Source: CAD feature listing. Evaluate the final solid. Frame: model axes, mm. Face numbers are marked on the shaded views. Give positions to 0.01 mm unless a question says otherwise; leave off trailing zeros. Order: outer loops, then holes, each group sorted by start corner. A loop starts at its lowest first (then second) coordinate and runs counter-clockwise, first axis right, second up. Notation, with made-up numbers: (66.5, 22.25) -> (121.5, 22.25) arc R21 ccw to (121.5, 30.25) -> close; hole circle Ø8 at (71.5, 57.5). An arc over 180 degrees is marked (long way). Answer in a Markdown table with one row per item.
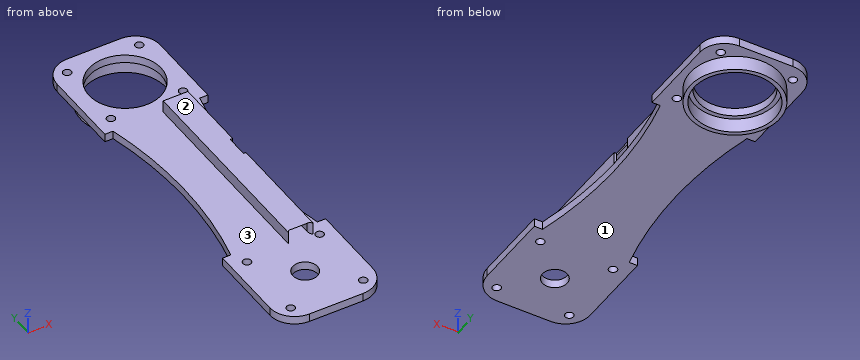
```python
from build123d import *

# Parameters (mm, degrees)
SKETCH1_R           = 11.1125
SKETCH1_R_2         = 1.27
BOSS_EXTRUDE1_DEPTH = 2.54
SKETCH2_R           = 1.27
SKETCH2_R_2         = 3.81
CUT_EXTRUDE1_DEPTH  = 2.54
SKETCH3_R           = 13.716
SKETCH3_R_2         = 12.446
BOSS_EXTRUDE2_DEPTH = 4.445
SKETCH4_W           = 7.62
SKETCH4_H           = 64.008
SKETCH4_W_2         = 6.096
SKETCH4_H_2         = 62.484
EXTRUDE_THIN1_DEPTH = 3.81
SKETCH5_W           = 6.096
SKETCH5_H           = 3.81
CUT_EXTRUDE2_DEPTH  = 76.2
SKETCH6_W           = 7.62
SKETCH6_H           = 64.008
BOSS_EXTRUDE3_DEPTH = 0.762
FILLET1_R           = 2.54
SKETCH7_W           = 3.81
SKETCH7_H           = 6.858
CUT_EXTRUDE3_DEPTH  = 0.762


with BuildPart() as part:
    # Sketch1 → Boss-Extrude1 (new body)
    with BuildSketch(Plane.XY):
        with BuildLine():
            Line((-13.335, -76.2), (-15.875, -76.2))
            Line((-15.875, -76.2), (-15.875, -100.33))
            ThreePointArc((-15.875, -100.33), (-13.643153673, -105.718153673), (-8.255, -107.95))
            Line((-8.255, -107.95), (8.255, -107.95))
            ThreePointArc((8.255, -107.95), (13.643153673, -105.718153673), (15.875, -100.33))
            Line((15.875, -100.33), (15.875, -76.2))
            Line((15.875, -76.2), (13.335, -76.2))
            ThreePointArc((13.335, -76.2), (9.716725547, -46.101), (13.335, -16.002))
            Line((13.335, -16.002), (15.875, -16.002))
            Line((15.875, -16.002), (15.875, 8.382))
            ThreePointArc((15.875, 8.382), (13.643153673, 13.770153673), (8.255, 16.002))
            Line((8.255, 16.002), (-8.255, 16.002))
            ThreePointArc((-8.255, 16.002), (-13.643153673, 13.770153673), (-15.875, 8.382))
            Line((-15.875, 8.382), (-15.875, -16.002))
            Line((-15.875, -16.002), (-13.335, -16.002))
            ThreePointArc((-13.335, -16.002), (-9.716725547, -46.101), (-13.335, -76.2))
        make_face()
        Circle(SKETCH1_R, mode=Mode.SUBTRACT)
        with Locations((11.1125, 11.2014)):
            Circle(SKETCH1_R_2, mode=Mode.SUBTRACT)
        with Locations((11.1125, -11.2014)):
            Circle(SKETCH1_R_2, mode=Mode.SUBTRACT)
        with Locations((-11.1125, -11.2014)):
            Circle(SKETCH1_R_2, mode=Mode.SUBTRACT)
        with Locations((-11.1125, 11.2014)):
            Circle(SKETCH1_R_2, mode=Mode.SUBTRACT)
    extrude(amount=BOSS_EXTRUDE1_DEPTH)

    # Sketch2 → Cut-Extrude1 (cut)
    with BuildSketch(Plane(origin=(0, 0, 0), x_dir=(-1, 0, 0), z_dir=(0, 0, -1))):
        with Locations((-11.176, -80.899)):
            Circle(SKETCH2_R)
        with Locations((11.176, -80.899)):
            Circle(SKETCH2_R)
        with Locations((11.176, -103.251)):
            Circle(SKETCH2_R)
        with Locations((-11.176, -103.251)):
            Circle(SKETCH2_R)
        with Locations((0, -92.075)):
            Circle(SKETCH2_R_2)
    extrude(amount=-CUT_EXTRUDE1_DEPTH, mode=Mode.SUBTRACT)

    # Sketch3 → Boss-Extrude2 (add)
    with BuildSketch(Plane(origin=(0, 0, 0), x_dir=(-1, 0, 0), z_dir=(0, 0, -1))):
        with Locations(Location((0, 0, 0), (0, 0, 180))):
            Circle(SKETCH3_R)
        Circle(SKETCH3_R_2, mode=Mode.SUBTRACT)
    extrude(amount=BOSS_EXTRUDE2_DEPTH)

    # Sketch4 → Extrude-Thin1 (add)
    with BuildSketch(Plane.XY.offset(2.54)):
        with Locations((5.906725547, -48.006)):
            Rectangle(SKETCH4_W, SKETCH4_H)
        with Locations((5.906725547, -48.006)):
            Rectangle(SKETCH4_W_2, SKETCH4_H_2, mode=Mode.SUBTRACT)
    extrude(amount=EXTRUDE_THIN1_DEPTH)

    # Sketch5 → Cut-Extrude2 (cut)
    with BuildSketch(Plane.XZ.offset(80.01)):
        with Locations((5.906725547, 4.445)):
            Rectangle(SKETCH5_W, SKETCH5_H)
    extrude(amount=-CUT_EXTRUDE2_DEPTH, mode=Mode.SUBTRACT)

    # Sketch6 → Boss-Extrude3 (add)
    with BuildSketch(Plane.XY.offset(6.35)):
        with Locations((5.906725547, -48.006)):
            Rectangle(SKETCH6_W, SKETCH6_H)
    extrude(amount=-BOSS_EXTRUDE3_DEPTH)

    # Fillet1
    # the kernel refuses this fillet: 2.54 mm, written as the material it takes off along each edge
    with BuildSketch(Plane(origin=(8.954725547, -80.01, 5.588), x_dir=(0, 1, 0), z_dir=(0, 0, -1)), Plane(origin=(2.858725547, -80.01, 2.54), x_dir=(0, 1, 0), z_dir=(0, 0, 1))) as fillet1_piece_1:
        with BuildLine():
            CenterArc((1.813922821, 2.54), FILLET1_R, 224.427004001, 45.572995999)
            Line((0, 0.762), (0, 0))
            Line((0, 0), (1.813922821, 0))
        make_face()
    extrude(amount=3.048, mode=Mode.SUBTRACT)
    with BuildSketch(Plane(origin=(8.954725547, -80.01, 5.588), x_dir=(0, 1, 0), z_dir=(-1, 0, 0))) as fillet1_piece_2:
        with BuildLine():
            CenterArc((FILLET1_R, -FILLET1_R), FILLET1_R, 90, 90)
            Line((0, -FILLET1_R), (0, 0))
            Line((0, 0), (FILLET1_R, 0))
        make_face()
    extrude(amount=6.096, mode=Mode.SUBTRACT)
    with BuildSketch(Plane(origin=(15.304725547, -80.01, 5.588), x_dir=(0, 1, 0), z_dir=(-1, 0, 0))) as fillet1_piece_3a_section:
        with BuildLine():
            CenterArc((FILLET1_R, -FILLET1_R), FILLET1_R, 90, 90)
            Line((0, -FILLET1_R), (0, 0))
            Line((0, 0), (FILLET1_R, 0))
        make_face()
    fillet1_piece_3a = extrude(amount=12.446, mode=Mode.PRIVATE)
    fillet1_piece_3a = split(fillet1_piece_3a, bisect_by=Plane(origin=(15.304725547, -80.01, 6.35), z_dir=(0, 0, -1)), keep=Keep.TOP, mode=Mode.PRIVATE)
    fillet1_piece_3a = split(fillet1_piece_3a, bisect_by=Plane(origin=(8.954725547, -80.01, 5.588), z_dir=(1, 0, 0)), keep=Keep.TOP, mode=Mode.PRIVATE)
    fillet1_piece_3a = split(fillet1_piece_3a, bisect_by=Plane(origin=(9.716725547, -80.01, 5.588), z_dir=(-1, 0, 0)), keep=Keep.TOP, mode=Mode.PRIVATE)
    with BuildSketch(Plane(origin=(8.954725547, -80.01, 10.122807052), x_dir=(0, 1, 0), z_dir=(0, 0, -1))) as fillet1_piece_3b_section:
        with BuildLine():
            CenterArc((1.813922821, 2.54), FILLET1_R, 224.427004001, 45.572995999)
            Line((0, 0.762), (0, 0))
            Line((0, 0), (1.813922821, 0))
        make_face()
    fillet1_piece_3b = extrude(amount=7.582807052, mode=Mode.PRIVATE)
    fillet1_piece_3b = split(fillet1_piece_3b, bisect_by=Plane(origin=(8.954725547, -80.01, 6.35), z_dir=(0, 0, -1)), keep=Keep.TOP, mode=Mode.PRIVATE)
    fillet1_piece_3b = split(fillet1_piece_3b, bisect_by=Plane(origin=(8.954725547, -80.01, 5.588), z_dir=(0, 0, 1)), keep=Keep.TOP, mode=Mode.PRIVATE)
    fillet1_piece_3 = fillet1_piece_3a & fillet1_piece_3b
    add(fillet1_piece_3, mode=Mode.SUBTRACT)
    with BuildSketch(Plane(origin=(2.858725547, -80.01, 2.54), x_dir=(0, 1, 0), z_dir=(0, 0, 1))) as fillet1_piece_4a_section:
        with BuildLine():
            CenterArc((1.813922821, 2.54), FILLET1_R, 224.427004001, 45.572995999)
            Line((0, 0.762), (0, 0))
            Line((0, 0), (1.813922821, 0))
        make_face()
    fillet1_piece_4a = extrude(amount=7.582807052, mode=Mode.PRIVATE)
    fillet1_piece_4a = split(fillet1_piece_4a, bisect_by=Plane(origin=(2.858725547, -80.01, 6.35), z_dir=(0, 0, -1)), keep=Keep.TOP, mode=Mode.PRIVATE)
    fillet1_piece_4a = split(fillet1_piece_4a, bisect_by=Plane(origin=(2.858725547, -80.01, 5.588), z_dir=(0, 0, 1)), keep=Keep.TOP, mode=Mode.PRIVATE)
    with BuildSketch(Plane(origin=(8.954725547, -80.01, 5.588), x_dir=(0, 1, 0), z_dir=(-1, 0, 0))) as fillet1_piece_4b_section:
        with BuildLine():
            CenterArc((FILLET1_R, -FILLET1_R), FILLET1_R, 90, 90)
            Line((0, -FILLET1_R), (0, 0))
            Line((0, 0), (FILLET1_R, 0))
        make_face()
    fillet1_piece_4b = extrude(amount=12.446, mode=Mode.PRIVATE)
    fillet1_piece_4b = split(fillet1_piece_4b, bisect_by=Plane(origin=(2.096725547, -80.01, 5.588), z_dir=(1, 0, 0)), keep=Keep.TOP, mode=Mode.PRIVATE)
    fillet1_piece_4b = split(fillet1_piece_4b, bisect_by=Plane(origin=(8.954725547, -80.01, 6.35), z_dir=(0, 0, -1)), keep=Keep.TOP, mode=Mode.PRIVATE)
    fillet1_piece_4b = split(fillet1_piece_4b, bisect_by=Plane(origin=(2.858725547, -80.01, 5.588), z_dir=(-1, 0, 0)), keep=Keep.TOP, mode=Mode.PRIVATE)
    fillet1_piece_4 = fillet1_piece_4a & fillet1_piece_4b
    add(fillet1_piece_4, mode=Mode.SUBTRACT)

    # Sketch7 → Cut-Extrude3 (cut)
    with BuildSketch(Plane(origin=(9.716725547, 0, 0), x_dir=(0, 0, -1), z_dir=(1, 0, 0))):
        with Locations((-4.445, -42.291)):
            Rectangle(SKETCH7_W, SKETCH7_H)
    extrude(amount=-CUT_EXTRUDE3_DEPTH, mode=Mode.SUBTRACT)


solid = part.part
```
(1) Pull-direction query (Z, two-part tool) for the marked faces 1, 2 and 3; classes: +Z half, -Z half, draft (parallel to the pull), parting line (faces both ways), or undercut.
A:
| item | result |
|---|---|
| face 1 | -Z half |
| face 2 | +Z half |
| face 3 | undercut |
(2) Section query B-B (y = 0). Return the cut outline in (x, z) (1 decimal), plus the area to 3 significant figures.
A:
| item | result |
|---|---|
| outline | (-15.9, 0) -> (-13.7, 0) -> (-13.7, -4.4) -> (-12.4, -4.4) -> (-12.4, 0) -> (-11.1, 0) -> (-11.1, 2.5) -> (-15.9, 2.5) -> close; (11.1, 0) -> (12.4, 0) -> (12.4, -4.4) -> (13.7, -4.4) -> (13.7, 0) -> (15.9, 0) -> (15.9, 2.5) -> (11.1, 2.5) -> close |
| area | 35.5 mm^2 |
(3) First-contact query: pin 1 Ø12 at (x, y) = (-12.5, -91) entering from +Z; pin 2 Ø3 at (x, z) = (15, 1) entering from +Y; pin 3 Ø1.5 at (x, z) = (8, 4) entering from -Y; pin 4 Ø1.1 at (y, z) = (-32.5, 4.5) entering from +X. Flat tips, straight axial feed; report the tip coordinate or a pass-through.
A:
| item | result |
|---|---|
| pin 1 | stops at z = 2.54 |
| pin 2 | stops at y = 13.91 |
| pin 3 | passes through |
| pin 4 | stops at x = 9.72 |
(4) Section query D-D (z = -1.75). Return the cut outline in (x, y), plus the area to 3 significant figures.
A:
| item | result |
|---|---|
| outline | circle Ø27.43 at (0, 0); hole circle Ø24.89 at (0, 0) |
| area | 104 mm^2 |
(5) Section query C-C (y = -67). Return the cut outline in (x, z), plus the area to 3 significant figures.
A:
| item | result |
|---|---|
| outline | (-11.45, 0) -> (11.45, 0) -> (11.45, 2.54) -> (9.72, 2.54) -> (9.72, 6.35) -> (2.1, 6.35) -> (2.1, 2.54) -> (-11.45, 2.54) -> close; hole (2.86, 2.54) -> (8.95, 2.54) -> (8.95, 5.59) -> (2.86, 5.59) -> close |
| area | 68.6 mm^2 |
(6) Section query A-A (x = 0). Give the number of separate pieces and of enclosed holes in the cut face, plus the area to 3 significant figures.
A:
| item | result |
|---|---|
| separate pieces | 3 |
| enclosed holes | 0 |
| area | 250 mm^2 |
(7) Ray query, probe 1 along X at (y, z) = (-82, 2) (3 decimals); probe 2 along Z at (x, y) = (6.5, -73); probe 3 along Y at (x, z) = (14, 2.5). Return the intervals inside material, ascending.
A:
| item | result |
|---|---|
| probe 1 | x = -15.875 to -11.809, -10.543 to 10.543, 11.809 to 15.875 |
| probe 2 | z = 0 to 2.54, 5.59 to 6.35 |
| probe 3 | y = -105.34 to -76.2, -16 to 13.39 |
